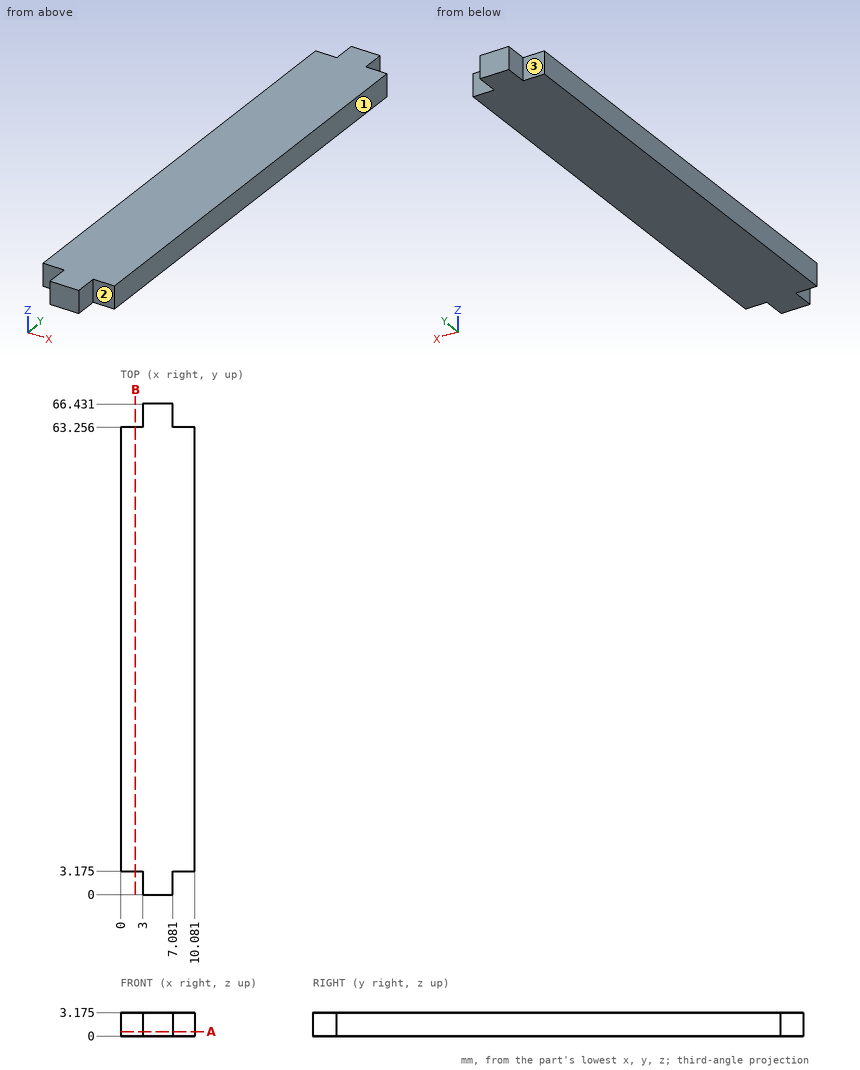
Could you check a few things on this drawing? It's one solid part, dimensions in mm from its lowest x, y, z. A direction names the side the tool comes from. Round coordinates to 2 decimals unless told otherwise and drop trailing zeros. Order: outer loops, then holes, each group sorted by start corner. A loop starts at its lowest first (then second) coordinate and runs counter-clockwise, first axis right, second up.
Q1. Imagine slicing it at A-A, the plane z = 0.6. List the corners of the cut face in (x, y) for me (1 decimal), then the cut area to 3 significant figures.
Geometry says:
outline: (0, 3.2) - (3, 3.2) - (3, 0) - (7.1, 0) - (7.1, 3.2) - (10.1, 3.2) - (10.1, 63.3) - (7.1, 63.3) - (7.1, 66.4) - (3, 66.4) - (3, 63.3) - (0, 63.3) - close
area: 632 mm2
Q2. Which directions (+Z, -Z, +X, -X, +Y, -Y) give clear straight access to the entire face, cutting with the end or side of a thin tool? Please do the marked faces 1, 2 and 3.
Geometry says:
face 1: +Z, -Z, +X, +Y, -Y
face 2: +Z, -Z, +X, -Y
face 3: +Z, -Z, -X, +Y
Q3. Imagine slicing it at B-B, the plane x = 2. List the corners of the cut face in (y, z) for me (1 decimal).
Geometry says:
outline: (3.2, 0) - (63.3, 0) - (63.3, 3.2) - (3.2, 3.2) - close
Q4. Please list where this line runs through material, in increasing order: probe 1 along Y at (x, z) = (2.75, 3.05) (1 decimal).
Geometry says:
probe 1: y = 3.2 to 63.3
Q5. I'm going to push flat-ended pins straight in: P1, Ø1.6, axis at y = 1, z = 1, coming from the +X side; P2, Ø1, axis at y = 1.5, z = 1.5, coming from the -X side; P3, Ø1, axis at x = 2, z = 2, coming from the +Y side; P4, Ø5, axis at x = 4, y = 8, coming from the -Z side. Where does each tip first touch, or does it pass through?
Geometry says:
P1: stops at x = 7.08
P2: stops at x = 3
P3: stops at y = 63.26
P4: stops at z = 0
